```python
from build123d import *

# Parameters (mm, degrees)
F0_R     = 37.5
F0_R_2   = 25
F1_DEPTH = 25
F2_DEPTH = 12.5
F3_R     = 10
F4_DEPTH = 85


with BuildPart() as f1:
    # F0 (on Top) → F1 (new body, symmetric)
    with BuildSketch(Plane.XY):
        Circle(F0_R)
        Circle(F0_R_2, mode=Mode.SUBTRACT)
    extrude(amount=F1_DEPTH, both=True)

    # F0 (on Top) → F2 (join, symmetric)
    with BuildSketch(Plane.XY):
        with BuildLine():
            Line((-45, 100), (-45, 0))
            ThreePointArc((-45, 0), (0, -45), (45, 0))
            Line((45, 0), (45, 100))
            Line((45, 100), (-45, 100))
        make_face()
        Circle(F0_R, mode=Mode.SUBTRACT)
    extrude(amount=F2_DEPTH, both=True)

    # F3 (on face) → F4 (join)
    with BuildSketch(Plane(origin=(0, 100, 0), x_dir=(-1, 0, 0), z_dir=(0, 1, 0))):
        Circle(F3_R)
    extrude(amount=F4_DEPTH)


solid = f1.part
```
Model file for the job. Use its own axes, mm. A direction names the side the tool comes from. Coordinates: 2 decimals unless noted, no trailing zeros. Order: outer loops, then holes, each group sorted by start corner. A loop starts at its lowest first (then second) coordinate and runs counter-clockwise, first axis right, second up. Notation, with made-up numbers: (37, 69) -> (54, 69) arc R18 cw to (54, 99) -> close; hole circle Ø3 at (33, -29). An arc over 180 degrees is marked (long way). Return JSON: item names as keys, results as strings.
Item 1: Slice it at A-A (x = 0). Write the cut outline in (y, z), then the cut area to 3 significant figures.
Model answer:
{"outline": "(-45, -12.5) -> (-37.5, -12.5) -> (-37.5, -25) -> (-25, -25) -> (-25, 25) -> (-37.5, 25) -> (-37.5, 12.5) -> (-45, 12.5) -> close; (25, -25) -> (37.5, -25) -> (37.5, -12.5) -> (100, -12.5) -> (100, -10) -> (185, -10) -> (185, 10) -> (100, 10) -> (100, 12.5) -> (37.5, 12.5) -> (37.5, 25) -> (25, 25) -> close", "area": "4,700 mm²"}
Item 2: Slice it at C-C (y = 9.5). Write the cut outline in (x, z).
Model answer:
{"outline": "(-45, -12.5) -> (-36.28, -12.5) -> (-36.28, -25) -> (-23.12, -25) -> (-23.12, 25) -> (-36.28, 25) -> (-36.28, 12.5) -> (-45, 12.5) -> close; (23.12, -25) -> (36.28, -25) -> (36.28, -12.5) -> (45, -12.5) -> (45, 12.5) -> (36.28, 12.5) -> (36.28, 25) -> (23.12, 25) -> close"}
Item 3: Slice it at D-D (x = 21.5). Write the cut outline in (y, z), then the cut area to 3 significant figures.
Model answer:
{"outline": "(-39.53, -12.5) -> (-30.72, -12.5) -> (-30.72, -25) -> (-12.76, -25) -> (-12.76, 25) -> (-30.72, 25) -> (-30.72, 12.5) -> (-39.53, 12.5) -> close; (12.76, -25) -> (30.72, -25) -> (30.72, -12.5) -> (100, -12.5) -> (100, 12.5) -> (30.72, 12.5) -> (30.72, 25) -> (12.76, 25) -> close", "area": "3,750 mm²"}
Item 4: Mould opens along X. For faces 4 (the face through (24, -8, -25)), 5 (the face through (23.846, 7.509, -0.35)), 6 (the face through (2.17, 141.9, -9.76)) say: pulls with the +X half, pulls with the -X half, needs draft (parallel to the pull), parting line crosses it, or undercut.
Model answer:
{"face 4": "needs draft", "face 5": "undercut", "face 6": "parting line crosses it"}
Item 5: 3-axis set-ups, long thin cutter, end or side, ignore diameter. For faces 1 (the face through (-4.88, 37.18, -18.66)), 2 (the face through (-4.88, 37.18, 18.84)), 3 (the face through (0, 185, 0)): which of +Z, -Z, +X, -X, +Y, -Y reach the whole face in a straight line?
Model answer:
{"face 1": "-Z", "face 2": "+Z", "face 3": "+Z, -Z, +X, -X, +Y"}
Item 6: Pin check, flat tips, straight feed: P1, Ø12, axis at x = 31.5, z = 11.5, coming from the -Y side; P2, Ø12, axis at y = 110, z = 14, coming from the -X side; P3, Ø2, axis at x = 27.5, z = 6, coming from the -Y side. Stop position of each tip, or through.
Model answer:
{"P1": "stops at y = -37.08", "P2": "stops at x = -6", "P3": "stops at y = -36.37"}
Item 7: Wall check: line 1 along Y through (x, z) = (0, 1); line 2 along Y through (x, z) = (0, -11); line 3 along Z through (x, y) = (-39, -12.5). Give the ranges that are in metal, low to high. Write a range as from..to.
Model answer:
{"line 1": "y = -45..-25, 25..185", "line 2": "y = -45..-25, 25..100", "line 3": "z = -12.5..12.5"}
Item 8: Slice it at B-B (z = 16). Write the cut outline in (x, y).
Model answer:
{"outline": "circle Ø75 at (0, 0); hole circle Ø50 at (0, 0)"}
